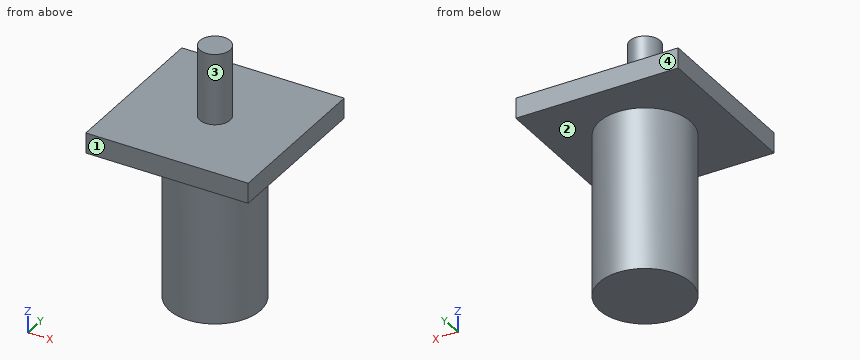
from build123d import *

# Parameters (mm, degrees)
F0_W     = 80
F0_H     = 80
F1_DEPTH = 10
F2_R     = 22.5
F3_DEPTH = 80
F4_R     = 7.5
F5_DEPTH = 35


with BuildPart() as f1:
    # F0 (on Top) → F1 (new body)
    with BuildSketch(Plane.XY):
        Rectangle(F0_W, F0_H)
    extrude(amount=-F1_DEPTH)

    # F2 (on face) → F3 (join)
    with BuildSketch(Plane(origin=(0, 0, -10), x_dir=(1, 0, 0), z_dir=(0, 0, -1))):
        Circle(F2_R)
    extrude(amount=F3_DEPTH)

    # F4 (on face) → F5 (join)
    with BuildSketch(Plane.XY):
        Circle(F4_R)
    extrude(amount=F5_DEPTH)


solid = f1.part
Model file for the job. Use its own axes, mm. Face numbers are marked on the shaded views. A direction names the side the tool comes from. Coordinates: 2 decimals unless noted, no trailing zeros. Write each loop counter-clockwise with the first axis right and the second up, starting at its lowest first coordinate (ties: lowest second). Pieces come first, ordered by that corner, then holes. Notation, with made-up numbers: (-4, -40) - (33, -40) arc R23 cw to (33, -1) - close; hole circle Ø11 at (-17.75, 54). An arc over 180 degrees is marked (long way). Write each question's results on one line, items separated by ' | '. Start each with the question number.
1) Mould opens along X. For the marked faces 3 and 4 say: pulls with the +X half, pulls with the -X half, needs draft (parallel to the pull), parting line crosses it, or undercut.
2) Cut at D-D (x = 19.5). Write the cut outline in (y, z), then the cut area to 3 significant figures.
3) Probe line 1 along Z through (x, y) = (3.5, 31.5); line 2 along Y through (x, z) = (0, 28); line 3 along Z through (x, y) = (-8.5, 19). List the from-to ranges inside material, lowest first. Write a range as from..to.
4) 3-axis set-ups, long thin cutter, end or side, ignore diameter. For the marked faces 1 and 2: which of +Z, -Z, +X, -X, +Y, -Y reach the whole face in a straight line?
5) Cut at A-A (y = 0). Write the cut outline in (x, z).
6) Cut at C-C (z = 22.5). Write the cut outline in (x, y), then the cut area to 3 significant figures.
7) Flat gauge pins, fed straight in: P1, Ø5, axis at y = 1.5, z = -40.5, coming from the +X side; P2, Ø5, axis at x = -1.5, z = -43.5, coming from the -Y side; P3, Ø1.5, axis at x = 19, y = -9.5, coming from the +Z side. Where does each tip first touch, or does it go through?
Returned:
1) face 3: parting line crosses it | face 4: needs draft
2) outline: (-40, -10) - (-11.22, -10) - (-11.22, -90) - (11.22, -90) - (11.22, -10) - (40, -10) - (40, 0) - (-40, 0) - close | area: 2,600 mm^2
3) line 1: -10..0 | line 2: -7.5..7.5 | line 3: -90..0
4) face 1: +Z, -Z, +X, -X, -Y | face 2: -Z
5) outline: (-40, -10) - (-22.5, -10) - (-22.5, -90) - (22.5, -90) - (22.5, -10) - (40, -10) - (40, 0) - (7.5, 0) - (7.5, 35) - (-7.5, 35) - (-7.5, 0) - (-40, 0) - close
6) outline: circle Ø15 at (0, 0) | area: 177 mm^2
7) P1: x = 22.5 | P2: y = -22.5 | P3: z = 0
